Verification items for the finished model (mm, model axes). Face numbers are marked on the shaded views. A direction names the side the tool comes from. Round coordinates to 2 decimals unless told otherwise and drop trailing zeros. Order: outer loops, then holes, each group sorted by start corner. A loop starts at its lowest first (then second) coordinate and runs counter-clockwise, first axis right, second up. Notation, with made-up numbers: M 62.25,57 L 72.25,57 A16 cw 72.25,78 Z; hole C 64,-37.5 d6. An arc over 180 degrees is marked long. Return JSON: item names as keys, results as strings. Group by question number.
from build123d import *

# Parameters (mm, degrees)
F0_W     = 20
F0_H     = 2
F1_DEPTH = 2.5
F0_W_2   = 25
F0_H_2   = 5
F2_DEPTH = 25
F4_DEPTH = 2.5
F0_W_3   = 2.5
F0_H_3   = 7
F5_DEPTH = 35
F6_DEPTH = 32.5
F7_DEPTH = 2.5


with BuildPart() as f1:
    # F0 (on Top) → F1 (new body)
    with BuildSketch(Plane.XY):
        Rectangle(F0_W, F0_H)
    extrude(amount=F1_DEPTH)

    # F0 (on Top) → F2 (join)
    with BuildSketch(Plane.XY):
        Rectangle(F0_W_2, F0_H_2)
        Rectangle(F0_W, F0_H, mode=Mode.SUBTRACT)
    extrude(amount=F2_DEPTH)

    # F3 (on face) → F4 (cut)
    with BuildSketch(Plane.XZ.offset(2.5)):
        with BuildLine():
            ThreePointArc((-8.75, 12.25), (0, 3.5), (8.75, 12.25))
            ThreePointArc((8.75, 12.25), (0, 21), (-8.75, 12.25))
        make_face()
        with BuildLine():
            ThreePointArc((-8.75, 12.25), (0, 21), (8.75, 12.25))
            Line((8.75, 12.25), (8.75, 25))
            Line((8.75, 25), (-8.75, 25))
            Line((-8.75, 25), (-8.75, 12.25))
        make_face()
    extrude(amount=-F4_DEPTH, mode=Mode.SUBTRACT)

    # F0 (on Top) → F5 (join)
    with BuildSketch(Plane.XY):
        Polygon((10, 12), (12.5, 12), (12.5, 14.5), (-12.5, 14.5), (-12.5, 12), (-10, 12), align=None)
        with Locations((-11.25, 8.5)):
            Rectangle(F0_W_3, F0_H_3)
        with Locations((0, 8.5)):
            Rectangle(F0_W, F0_H_3)
        Polygon((-12.5, 2.5), (12.5, 2.5), (12.5, 5), (10, 5), (-10, 5), (-12.5, 5), align=None)
        with Locations((11.25, 8.5)):
            Rectangle(F0_W_3, F0_H_3)
    extrude(amount=F5_DEPTH)

    # F0 (on Top) → F6 (cut)
    with BuildSketch(Plane.XY):
        with Locations((11.25, 8.5)):
            Rectangle(F0_W_3, F0_H_3)
        with Locations((0, 8.5)):
            Rectangle(F0_W, F0_H_3)
        with Locations((-11.25, 8.5)):
            Rectangle(F0_W_3, F0_H_3)
    extrude(amount=F6_DEPTH, mode=Mode.SUBTRACT)

    # F0 (on Top) → F7 (join)
    with BuildSketch(Plane.XY):
        with Locations((11.25, 8.5)):
            Rectangle(F0_W_3, F0_H_3)
        with Locations((0, 8.5)):
            Rectangle(F0_W, F0_H_3)
        with Locations((-11.25, 8.5)):
            Rectangle(F0_W_3, F0_H_3)
        Polygon((10, 12), (12.5, 12), (12.5, 14.5), (-12.5, 14.5), (-12.5, 12), (-10, 12), align=None)
        Polygon((-12.5, 2.5), (12.5, 2.5), (12.5, 5), (10, 5), (-10, 5), (-12.5, 5), align=None)
    extrude(amount=F7_DEPTH)


solid = f1.part
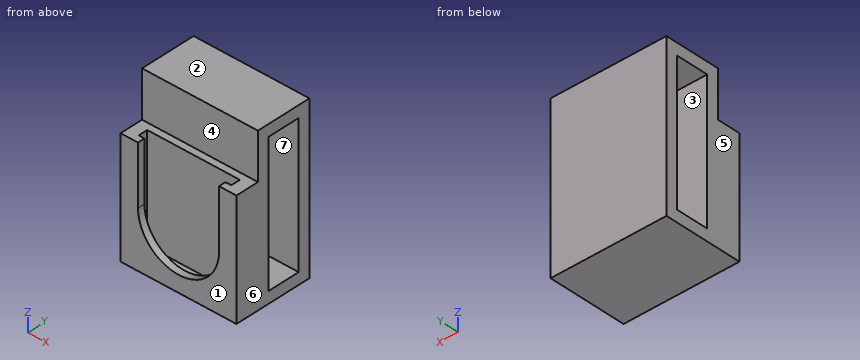
1. Cross-section at D-D (x = -3). Enter the section's corners in (y, z), plus the area to 3 significant figures.
2. Draft check along Y on the marked faces 1, 2 and 3. Enter one of: +Y half, -Y half, draft (parallel to the pull), parting line (faces both ways), or undercut.
3. Cross-section at B-B (x = 0). Enter the section's corners in (y, z), plus the area to 3 significant figures.
4. Go/stop test with flat-tipped pins: pin 1 (1.5 mm diameter, centred on x = -2, y = -0.5, fed in from +Z); pin 2 (11 mm diameter, centred on x = -1.5, z = 31, fed in from -Y); pin 3 (6 mm diameter, centred on x = -4.5, z = 16, fed in from -Y); pin 4 (5 mm diameter, centred on x = -4.5, y = 3, fed in from -Z). Record where each tip stops, or that it passes through.
5. Cross-section at C-C (z = 26.5). Enter the section's corners in (x, y), plus the area to 3 significant figures.
6. Thickness scan on line 1 along Y through (x, z) = (-9, 16); line 2 along X through (y, z) = (0.75, 3); line 3 along Y through (x, z) = (1.75, 16). Record the ranges inside material, lowest first. Write a range as from..to.
7. Cross-section at A-A (z = 16.5). Enter the section's corners in (x, y).
8. Access from +Z, -Z, +X, -X, +Y, -Y to the whole of each face (thin tool, end or side, straight path). Record for the marked faces 4, 5, 6 and 7.
Computed:
{
 "1": {"outline": "M -2.5,0 L 14.5,0 L 14.5,35 L 2.5,35 L 2.5,25 L 1,25 L 1,2.5 L -1,2.5 L -1,4.03 L -2.5,4.03 Z; hole M 5,2.5 L 12,2.5 L 12,32.5 L 5,32.5 Z", "area": "259 mm²"},
 "2": {"face 1": "-Y half", "face 2": "draft", "face 3": "undercut"},
 "3": {"outline": "M -2.5,0 L 14.5,0 L 14.5,35 L 2.5,35 L 2.5,25 L 1,25 L 1,2.5 L -1,2.5 L -1,3.5 L -2.5,3.5 Z; hole M 5,2.5 L 12,2.5 L 12,32.5 L 5,32.5 Z", "area": "258 mm²"},
 "4": {"pin 1": "stops at z = 3.88", "pin 2": "stops at y = 2.5", "pin 3": "stops at y = 1", "pin 4": "stops at z = 0"},
 "5": {"outline": "M -12.5,2.5 L 12.5,2.5 L 12.5,5 L -12.5,5 Z; M -12.5,12 L 12.5,12 L 12.5,14.5 L -12.5,14.5 Z", "area": "125 mm²"},
 "6": {"line 1": "y = -2.5..-1, 1..5, 12..14.5", "line 2": "x = -12.5..-10, 10..12.5", "line 3": "y = 1..5, 12..14.5"},
 "7": {"outline": "M -12.5,-2.5 L -8.75,-2.5 L -8.75,-1 L -10,-1 L -10,1 L 10,1 L 10,-1 L 8.75,-1 L 8.75,-2.5 L 12.5,-2.5 L 12.5,5 L -12.5,5 Z; M -12.5,12 L 12.5,12 L 12.5,14.5 L -12.5,14.5 Z"},
 "8": {"face 4": "+Z, +X, -X, -Y", "face 5": "+Z, -Z, -X, +Y, -Y", "face 6": "+Z, -Z, +X, +Y, -Y", "face 7": "+X, -X"}
}
